Source: CAD feature listing. Evaluate the final solid. Frame: model axes, mm. Face numbers are marked on the shaded views. Coordinates: 2 decimals unless noted, no trailing zeros. Order: outer loops, then holes, each group sorted by start corner. A loop starts at its lowest first (then second) coordinate and runs counter-clockwise, first axis right, second up. Notation, with made-up numbers: (61, -22) -> (88, -22) arc R13 cw to (88, -12) -> close; hole circle Ø4 at (60.25, 36.25). An arc over 180 degrees is marked (long way). Write item = value, one per line. Start each with the question number.
Item 1: Section query D-D (x = 7.5). Output: boundary loops of the cut face in (y, z).
Item 2: Mould query, pull axis X, two halves, no side actions, for the marked faces 1, 2 and 3. Classes: released by +X, released by -X, zero draft, split by the parting line, or undercut.
Item 3: Section query C-C (x = -11.75). Output: boundary loops of the cut face in (y, z), then the cut area to 3 significant figures.
Item 4: Ray query, line 1 along X through (y, z) = (0, -28); line 2 along Z through (x, y) = (-1.75, -7.75); line 3 along Y through (x, z) = (0, 13). Return the intervals inside material, ascending. Write a range as [from, to].
Item 5: Section query B-B (y = -11). Output: boundary loops of the cut face in (x, z), then the cut area to 3 significant figures.
Item 6: Section query A-A (x = 1.75). Output: boundary loops of the cut face in (y, z).
Item 7: Contact query for flat-ended pins moving along their axis: pin 1 (1.5 mm diameter, centred on y = -11.5, z = -27, fed in from +X); pin 2 (10 mm diameter, centred on x = 7, z = -0.5, fed in from -Y); pin 3 (1.5 mm diameter, centred on y = -11.5, z = 16, fed in from -X). Output: stop coordinate, or through.
```python
from build123d import *

# Parameters (mm, degrees)
F2_ANGLE = 320


with BuildPart() as f2:
    # F0 (on Front) → F2 (revolve, symmetric)
    with BuildSketch(Plane.XZ) as f2_sk:
        Polygon((0, 36.260698), (0, 38.260698), (-15, 38.260698), (-15, -46.739302), (-13, -46.739302), (-13, 36.260698), align=None)
    revolve(axis=Axis((0, 0, -8.945528), (0, 0, -1)), revolution_arc=F2_ANGLE / 2)
    revolve(f2_sk.sketch, axis=Axis((0, 0, -8.945528), (0, 0, 1)), revolution_arc=F2_ANGLE / 2)


solid = f2.part
```
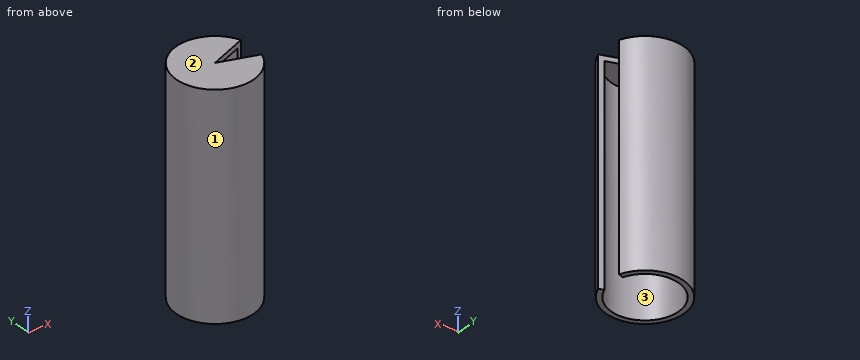
Computed:
q1.outline = (-12.99, -46.74) -> (-10.62, -46.74) -> (-10.62, 36.26) -> (-2.73, 36.26) -> (-2.73, 38.26) -> (-12.99, 38.26) -> close; (2.73, 36.26) -> (10.62, 36.26) -> (10.62, -46.74) -> (12.99, -46.74) -> (12.99, 38.26) -> (2.73, 38.26) -> close
q2.face_1 = split by the parting line
q2.face_2 = zero draft
q2.face_3 = undercut
q3.outline = (-9.32, -46.74) -> (-5.56, -46.74) -> (-5.56, 36.26) -> (5.56, 36.26) -> (5.56, -46.74) -> (9.32, -46.74) -> (9.32, 38.26) -> (-9.32, 38.26) -> close
q3.area = 662 mm^2
q4.line_1 = [-15, -13]
q4.line_2 = [36.26, 38.26]
q4.line_3 = [-15, -13], [13, 15]
q5.outline = (-10.2, -46.74) -> (-6.93, -46.74) -> (-6.93, 36.26) -> (6.93, 36.26) -> (6.93, -46.74) -> (10.2, -46.74) -> (10.2, 38.26) -> (-10.2, 38.26) -> close
q5.area = 584 mm^2
q6.outline = (-14.9, -46.74) -> (-12.88, -46.74) -> (-12.88, 36.26) -> (-0.64, 36.26) -> (-0.64, 38.26) -> (-14.9, 38.26) -> close; (0.64, 36.26) -> (12.88, 36.26) -> (12.88, -46.74) -> (14.9, -46.74) -> (14.9, 38.26) -> (0.64, 38.26) -> close
q7.pin_1 = 10.46
q7.pin_2 = -14.87
q7.pin_3 = -10.46
